Design review of the part shown in the three views and the two pictorial views. Dimensions are in mm from the part's minimum x, y and z. Coordinates: 2 decimals unless noted, no trailing zeros. Loops run counter-clockwise (first coordinate to the right, second up) from the corner with the lowest first, then second, coordinate; pieces in that order, holes last. Notation, with made-up numbers: M 63.5,61 L 120.5,61 A13 ccw 120.5,79 Z; hole C 65.25,86 d6. An arc over 180 degrees is marked long. Answer as a JSON object with one key per item and string values. Group by question number.
Item 1: Mouldability with a two-part tool opening along Y and no side actions: class the marked faces 1, 2, 3 and 4 as +Y half, -Y half, draft (parallel to the pull), parting line (faces both ways), or undercut.
Item 2: Add section A-A (x = 22.75). State the section outline as (y, z) points, then the cut area to 3 significant figures.
Item 3: Insertion check: pin 1 (5 mm diameter, centred on y = 22, z = 23, fed in from +X). The pin has a flat end and moves straight along its axis. Give the tip position at first contact, or say it passes through.
Item 4: Add section C-C (z = 208.5). State the section outline as (x, y) points, then the cut area to 3 significant figures.
Item 5: Wall thickness on L1, parallel to X at y = 6.5, z = 104; L2, parallel to Y at x = 7, z = 96.5; L3, parallel to Y at x = 27, z = 144: over which ranges is each line inside the solid? List them lowest first. Write a range as from..to.
Item 6: Add section D-D (y = 34.5). State the section outline as (x, z) points, then the cut area to 3 significant figures.
Item 7: Add section B-B (y = 50.5). State the section outline as (x, z) points.
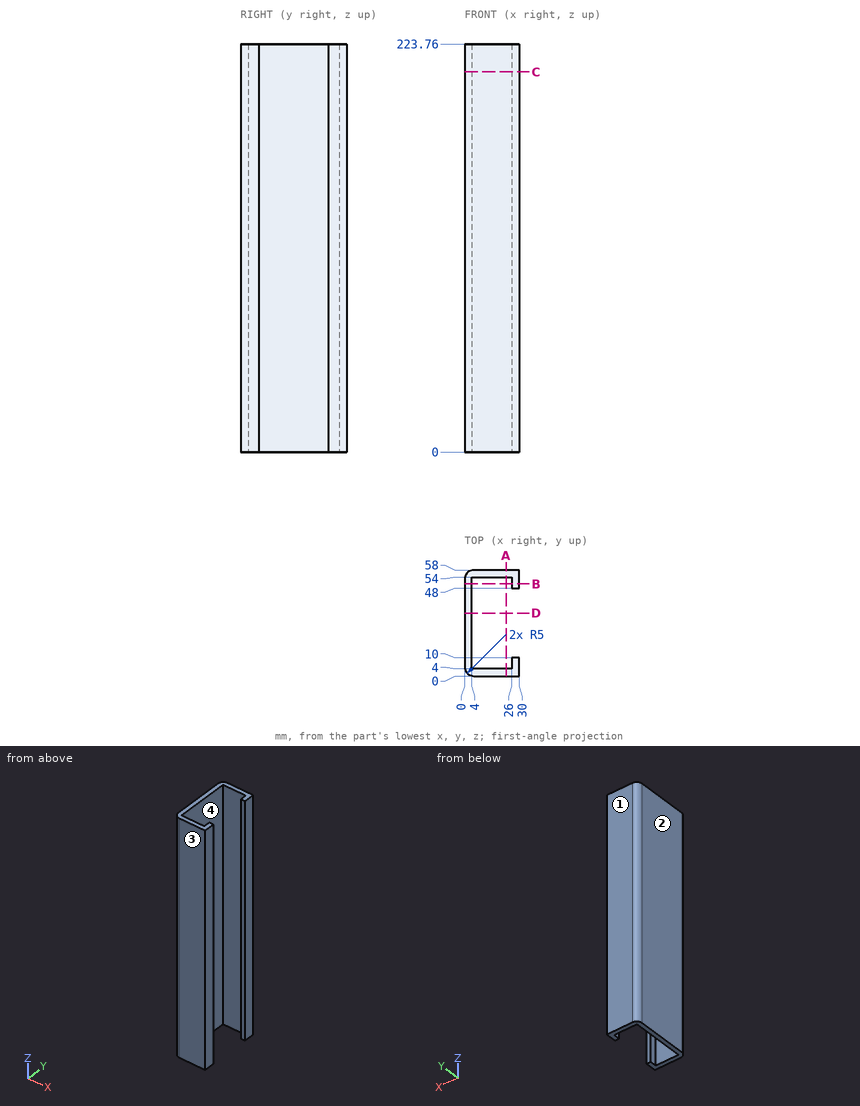
From the geometry:
{
 "1": {"face 1": "+Y half", "face 2": "draft", "face 3": "-Y half", "face 4": "undercut"},
 "2": {"outline": "M 0,0 L 4,0 L 4,223.76 L 0,223.76 Z; M 54,0 L 58,0 L 58,223.76 L 54,223.76 Z", "area": "1,790 mm²"},
 "3": {"pin 1": "stops at x = 4"},
 "4": {"outline": "M 0,5 A5 ccw 5,0 L 30,0 L 30,10 L 26,10 L 26,4 L 4,4 L 4,54 L 26,54 L 26,48 L 30,48 L 30,58 L 5,58 A5 ccw 0,53 Z", "area": "477 mm²"},
 "5": {"L1": "x = 0..4, 26..30", "L2": "y = 0..4, 54..58", "L3": "y = 0..10, 48..58"},
 "6": {"outline": "M 0,0 L 4,0 L 4,223.76 L 0,223.76 Z", "area": "895 mm²"},
 "7": {"outline": "M 0,0 L 4,0 L 4,223.76 L 0,223.76 Z; M 26,0 L 30,0 L 30,223.76 L 26,223.76 Z"}
}
